```python
from build123d import *

# Parameters (mm, degrees)
BOSS_EXTRUDE1_DEPTH = 25.4
SKETCH2_OUTSIDE_W   = 27.54
SKETCH2_OUTSIDE_H   = 25.576
SKETCH2_OUTSIDE_R   = 6.35
CUT_EXTRUDE2_DEPTH  = 7.9502
SKETCH3_OUTSIDE_W   = 27.54
SKETCH3_OUTSIDE_H   = 25.576
SKETCH3_OUTSIDE_R   = 6.875
CUT_EXTRUDE4_DEPTH  = 52.717751627
SKETCH4_R           = 2.0193
CUT_EXTRUDE5_DEPTH  = 52.654894492


with BuildPart() as part:
    # Sketch1 → Boss-Extrude1 (new, symmetric)
    with BuildSketch(Plane.XY):
        Polygon((7.332348419, 0), (3.666174209, 6.35), (-3.666174209, 6.35), (-7.332348419, 0), (-3.666174209, -6.35), (3.666174209, -6.35), align=None)
    extrude(amount=BOSS_EXTRUDE1_DEPTH, both=True)

    # Sketch2 outside → Cut-Extrude2 (cut)
    with BuildSketch(Plane.XY.offset(25.4)):
        Rectangle(SKETCH2_OUTSIDE_W, SKETCH2_OUTSIDE_H)
        Circle(SKETCH2_OUTSIDE_R, mode=Mode.SUBTRACT)
    cut_extrude2 = extrude(amount=-CUT_EXTRUDE2_DEPTH, mode=Mode.SUBTRACT)

    # Sketch3 outside → Cut-Extrude4 (cut, through all)
    with BuildSketch(Plane.XY.offset(25.4)):
        Rectangle(SKETCH3_OUTSIDE_W, SKETCH3_OUTSIDE_H)
        Circle(SKETCH3_OUTSIDE_R, mode=Mode.SUBTRACT)
    extrude(amount=-CUT_EXTRUDE4_DEPTH, mode=Mode.SUBTRACT)

    # Mirror1: Cut-Extrude2 across plane
    add(cut_extrude2.mirror(Plane.XY), mode=Mode.SUBTRACT)

    # Sketch4 → Cut-Extrude5 (cut, through all)
    with BuildSketch(Plane.XY.offset(25.4)):
        Circle(SKETCH4_R)
    extrude(amount=-CUT_EXTRUDE5_DEPTH, mode=Mode.SUBTRACT)


solid = part.part
```
Model file for the job. Use its own axes, mm. A direction names the side the tool comes from. Coordinates: 2 decimals unless noted, no trailing zeros. Order: outer loops, then holes, each group sorted by start corner. A loop starts at its lowest first (then second) coordinate and runs counter-clockwise, first axis right, second up. Notation, with made-up numbers: (16.5, 75.25) -> (60.5, 75.25) arc R15 ccw to (60.5, 89.25) -> close; hole circle Ø3 at (-17.75, -19.5). An arc over 180 degrees is marked (long way). Return JSON: item names as keys, results as strings.
Item 1: Wall check: line 1 along Y through (x, z) = (-1.75, -14.5); line 2 along X through (y, z) = (-0.25, -16.5); line 3 along Y through (x, z) = (-0.5, 6). Give the ranges that are in metal, low to high. Write a range as from..to.
Model answer:
{"line 1": "y = -6.35..-1.01, 1.01..6.35", "line 2": "x = -6.87..-2, 2..6.87", "line 3": "y = -6.35..-1.96, 1.96..6.35"}
Item 2: Slice it at A-A (y = 0). Write the cut outline in (x, z) (3 decimals), then the cut area to 3 significant figures.
Model answer:
{"outline": "(-6.875, -17.45) -> (-6.35, -17.45) -> (-6.35, -25.4) -> (-2.019, -25.4) -> (-2.019, 25.4) -> (-6.35, 25.4) -> (-6.35, 17.45) -> (-6.875, 17.45) -> close; (2.019, -25.4) -> (6.35, -25.4) -> (6.35, -17.45) -> (6.875, -17.45) -> (6.875, 17.45) -> (6.35, 17.45) -> (6.35, 25.4) -> (2.019, 25.4) -> close", "area": "477 mm²"}
Item 3: Mould opens along X. For faces 1 (the face through (-6.5, 0, 17.45)), 2 (the face through (5.52, 3.14, 0.24)), 3 (the face through (1.926, 0.607, 0.356)) say: pulls with the +X half, pulls with the -X half, needs draft (parallel to the pull), parting line crosses it, or undercut.
Model answer:
{"face 1": "needs draft", "face 2": "pulls with the +X half", "face 3": "undercut"}
Item 4: Slice it at B-B (z = -5). Write the cut outline in (x, y) (3 decimals).
Model answer:
{"outline": "(-6.817, -0.893) -> (-4.182, -5.457) arc R6.875 ccw to (-2.635, -6.35) -> (2.635, -6.35) arc R6.875 ccw to (4.182, -5.457) -> (6.817, -0.893) arc R6.875 ccw to (6.817, 0.893) -> (4.182, 5.457) arc R6.875 ccw to (2.635, 6.35) -> (-2.635, 6.35) arc R6.875 ccw to (-4.182, 5.457) -> (-6.817, 0.893) arc R6.875 ccw to start; hole circle Ø4.039 at (0, 0)"}
Item 5: Slice it at D-D (y = -2.5). Write the cut outline in (x, z), then the cut area to 3 significant figures.
Model answer:
{"outline": "(-5.89, -17.45) -> (-5.84, -17.45) -> (-5.84, -25.4) -> (5.84, -25.4) -> (5.84, -17.45) -> (5.89, -17.45) -> (5.89, 17.45) -> (5.84, 17.45) -> (5.84, 25.4) -> (-5.84, 25.4) -> (-5.84, 17.45) -> (-5.89, 17.45) -> close", "area": "597 mm²"}
Item 6: 3-axis set-ups, long thin cutter, end or side, ignore diameter. For faces 4 (the face through (6.5, 0, -17.45)), 5 (the face through (3, 6, 17.45)), 6 (the face through (3, 6, -17.45)): which of +Z, -Z, +X, -X, +Y, -Y reach the whole face in a straight line?
Model answer:
{"face 4": "-Z, +X", "face 5": "+Z, +X, +Y", "face 6": "-Z, +X, +Y"}
Item 7: Pin check, flat tips, straight feed: P1, Ø6.5, axis at x = 0, y = 0, coming from the -Z side; P2, Ø2, axis at x = 2, z = 18.5, coming from the -Y side; P3, Ø3, axis at y = -3, z = -17, coming from the -X side; P4, Ø3, axis at y = -4.5, z = -3, coming from the +X side. Stop position of each tip, or through.
Model answer:
{"P1": "stops at z = -25.4", "P2": "stops at y = -6.27", "P3": "stops at x = -6.47", "P4": "stops at x = 5.6"}
